Autodesk Inventor part; units mm, degrees
ref_plane "YZ Plane" through (0, 0, 0) normal (1, 0, 0) x (0, 1, 0)
ref_plane "XZ Plane" through (0, 0, 0) normal (0, 1, 0) x (-1, 0, 0)
ref_plane "XY Plane" through (0, 0, 0) normal (0, 0, 1) x (1, 0, 0)
sketch "Sketch1" plane through (0, 0, 0) normal (0, 0, 1) x (1, 0, 0)
  line L0 (23.2261, 43.4376) -> (23.2261, 3.4376)
  line L1 (23.2261, 43.4376) -> (93.2261, 43.4376)
  line L2 (93.2261, 43.4376) -> (93.2261, 3.4376)
  line L3 (93.2261, 3.4376) -> (23.2261, 3.4376)
  line L4 (23.2261, 3.4376) -> (93.2261, 13.4376)
  line L5 (58.2261, 8.4376) -> (58.2261, 3.4376)
  line L6 (98.2261, 48.4376) -> (18.2261, 48.4376)
  line L7 (18.2261, 48.4376) -> (18.2261, -1.5624)
  line L8 (18.2261, -1.5624) -> (98.2261, -1.5624)
  line L9 (98.2261, -1.5624) -> (98.2261, 48.4376)
  line L10 (23.2261, 43.4376) -> (23.2261, 48.4376)
  line L11 (93.2261, 43.4376) -> (93.2261, 48.4376)
  line L12 (58.2261, 43.4376) -> (58.2261, 48.4376)
  point P0 (0, 0)
  dimension "d0" = 40
  dimension "d1" = 70
  dimension "d2" = 10
  dimension "d4" = 5
  dimension "d5" = 5
  dimension "d16" = 35
extrude "Extrusion1" add sketch "Sketch1" along normal blind 60 contours L10 L6 L12 L1 | L0 L3 L2 L11 L6 L9 L8 L7 L10
extrude "Extrusion2" add sketch "Sketch1" along normal blind 5 contours L1 L2 L4 L0
extrude "Extrusion3" add sketch "Sketch1" along normal blind 60 contours L5 L4 L2 L3
sketch "Sketch2" plane through (18.2261, -1.5624, 0) normal (-1, 0, 0) x (0, 0, 1)
  line L0 (60, 0) -> (60, 50)
  line L1 (60, 0) -> (60, 5)
  line L2 (5, 10) -> (60, 10)
  line L3 (60, 5) -> (5, 10)
  line L4 (5, 5) -> (5, 45)
  line L5 (5, 5) -> (5, 10)
  line L6 (5, 5) -> (60, 5)
  point P0 (0, 1.5624)
  dimension "d12" = 5
extrude "Extrusion4" add sketch "Sketch2" against normal blind 45 contours L6 L4 L3
sketch "Sketch3" plane through (0, 0, 60) normal (0, 0, 1) x (1, 0, 0)
  line L0 (18.2261, 48.4376) -> (18.2261, -1.5624)
  line L1 (18.2261, -1.5624) -> (98.2261, -1.5624)
  line L2 (18.2261, 48.4376) -> (98.2261, 48.4376)
  line L3 (98.2261, 48.4376) -> (98.2261, -1.5624)
  line L4 (98.2261, -1.5624) -> (18.2261, -1.5624)
  line L5 (18.2261, -1.5624) -> (18.2261, 48.4376)
  point P0 (0, 0)
extrude "Extrusion5" add sketch "Sketch3" against normal blind 5
sketch "Sketch4" plane through (18.2261, -1.5624, 0) normal (0, -1, 0) x (1, 0, 0)
  line L0 (0, 0) -> (0, 60)
  line L1 (0, 60) -> (40, 60)
  line L2 (40, 60) -> (40, 25)
  line L3 (40, 25) -> (0, 25)
  line L4 (0, 25) -> (0, 60)
  line L5 (5, 55) -> (5, 5)
  line L6 (5, 25) -> (5, 55)
  line L7 (5, 55) -> (40, 55)
  point P0 (-18.2261, 0)
  point P1 (0, 25)
  dimension "d19" = 40
  dimension "d20" = 35
extrude "Extrusion6" cut sketch "Sketch4" against normal blind 10 contours L5 L7 L2 L3
properties part number "leftcollection"
Read the model definition and answer for the solid it produces. Units are mm, in the model's axes. A direction names the side the tool comes from. Give positions to 0.01 mm unless a question says otherwise; leave off trailing zeros. Order: outer loops, then holes, each group sorted by start corner. A loop starts at its lowest first (then second) coordinate and runs counter-clockwise, first axis right, second up. Notation, with made-up numbers: (56, 85) -> (96, 85) arc R15 ccw to (96, 90) -> close; hole circle Ø9 at (46, 38.5). An arc over 180 degrees is marked (long way). One line per item, written item: value. Start each with the question number.
(1) Flat-ended cylindrical pins translate along their axes: P1, Ø1.5, axis at x = 79.5, z = 1.5, coming from the +Y side; P2, Ø3, axis at x = 73, z = 40.5, coming from the +Y side; P3, Ø10, axis at x = 71.5, z = 18, coming from the +Y side. Find the tip coordinate at first contact, or state that the pin passes through.
(2) The part is cut by section C-C (x = 35). Determine the outline of the cut face in (y, z).
(3) A tool of negligible diameter and unlimited length cuts with its end or side. For faces 1 (the flat face through (41, 2, 25)), 2 (the flat face through (75, 43.438, 2)), 3 (the flat face through (58.226, 6, 2)), 4 (the flat face through (93.226, 31, 27)), 5 (the flat face through (58, 26, 5)), from which of +Z, -Z, +X, -X, +Y, -Y can it reach the whole face along a straight path? Write none if from no direction.
(4) The part is cut by section D-D (z = 7). Determine the outline of the cut face in (x, y), and give its area (3 significant figures).
(5) For a pull along X with two mould halves and no side action, classify faces 6 (the flat face through (40.481, 5.903, 2.465)), 7 (the flat face through (58, -1.562, 23)), 8 (the flat face through (98.226, 23, 30)) as released by +X, released by -X, zero draft, split by the parting line, or undercut.
(6) The part is cut by section A-A (y = 31.5). Determine the outline of the cut face in (x, z), and give its area (3 significant figures).
(7) The part is cut by section B-B (z = 38.5). Determine the outline of the cut face in (x, y).
(8) Straight lines are drawn through the part: L1, parallel to X at y = 1.5, z = 27.5; L2, parallel to X at y = 44, z = 18; L3, parallel to Z at x = 41, y = 24. For each, find the intervals that lie inside material, in ascending order.
Taken from the geometry:
1. P1: y = 43.44
1. P2: y = 10.76
1. P3: y = 11.05
2. outline: (-1.56, 0) -> (3.44, 0) -> (3.44, 5) -> (5.12, 5) -> (5.12, 0) -> (48.44, 0) -> (48.44, 60) -> (-1.56, 60) -> (-1.56, 55) -> (43.44, 55) -> (43.44, 5) -> (8.44, 5) -> (6.62, 25) -> (-1.56, 25) -> close
3. face 1: -Y
3. face 2: -Z, +Y
3. face 3: -Z
3. face 4: +Y
3. face 5: none
4. outline: (18.23, -1.56) -> (98.23, -1.56) -> (98.23, 48.44) -> (93.23, 48.44) -> (93.23, 13.44) -> (58.23, 8.44) -> (58.23, 8.26) -> (23.23, 8.26) -> (23.23, 43.44) -> (58.23, 43.44) -> (58.23, 48.44) -> (18.23, 48.44) -> close
4. area: 1,460 mm^2
5. face 6: undercut
5. face 7: zero draft
5. face 8: released by +X
6. outline: (18.23, 0) -> (98.23, 0) -> (98.23, 60) -> (18.23, 60) -> close; hole (23.23, 5) -> (93.23, 5) -> (93.23, 55) -> (23.23, 55) -> close
6. area: 1,300 mm^2
7. outline: (18.23, -1.56) -> (23.23, -1.56) -> (23.23, 43.44) -> (58.23, 43.44) -> (58.23, 48.44) -> (18.23, 48.44) -> close; (58.23, -1.56) -> (98.23, -1.56) -> (98.23, 48.44) -> (93.23, 48.44) -> (93.23, 13.44) -> (58.23, 8.44) -> close
8. L1: 18.23 to 23.23, 58.23 to 98.23
8. L2: 18.23 to 58.23, 93.23 to 98.23
8. L3: 0 to 5, 55 to 60
